Design review of the part shown in the three views and the two pictorial views. Dimensions are in mm from the part's minimum x, y and z. Round coordinates to 2 decimals unless told otherwise and drop trailing zeros. Write each loop counter-clockwise with the first axis right and the second up, starting at its lowest first coordinate (ties: lowest second). Pieces come first, ordered by that corner, then holes. Notation, with made-up numbers: (77, 29.25) - (128, 29.25) arc R21 ccw to (128, 68.25) - close; hole circle Ø5 at (-16.75, 6.25). An arc over 180 degrees is marked (long way). Use one line per item in the form item = value.
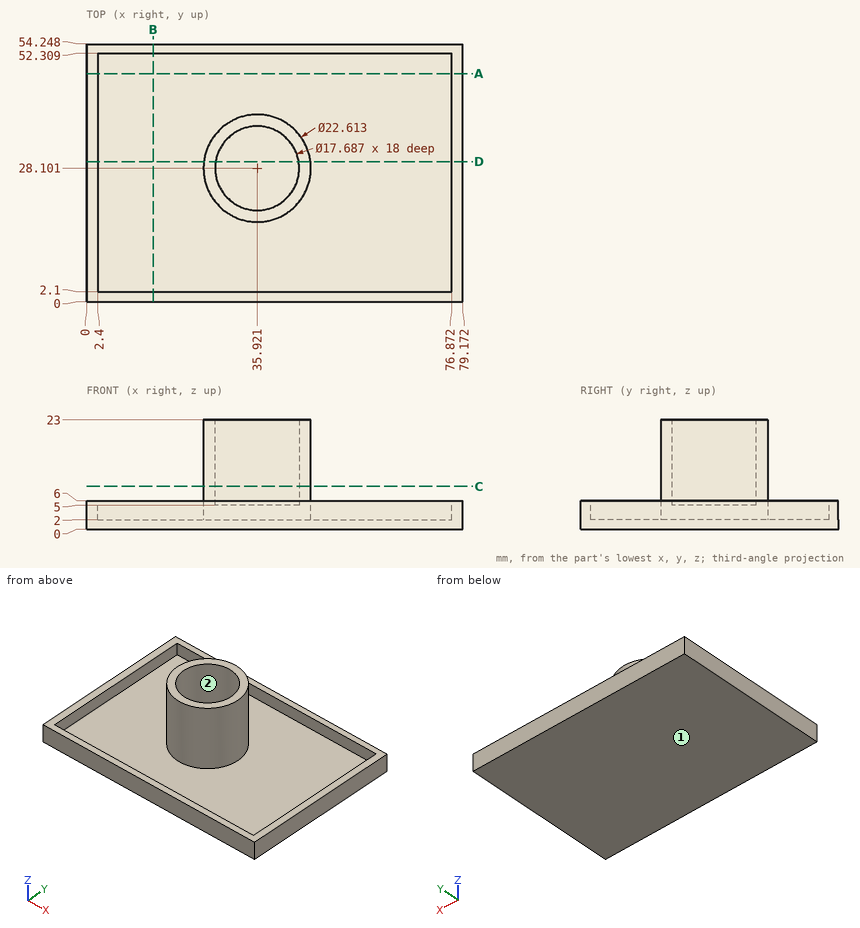
Q1. Draft analysis for pull direction X (two halves, no side actions). For the marked faces 1 and 2, state which applies: released by +X, released by -X, zero draft, split by the parting line, or undercut.
Calculated:
face_1 = zero draft
face_2 = undercut
Q2. To check wall thickness, follow line 1 along X through (y, z) = (28, 19.25) (1 decimal); line 2 along X through (y, z) = (47, 5.75); line 3 along Y through (x, z) = (66, 5). State the ranges of each line that lie inside material, in increasing order. Write a range as from..to.
Calculated:
line_1 = 24.6..27.1, 44.8..47.2
line_2 = 0..2.4, 76.87..79.17
line_3 = 0..2.1, 52.31..54.25
Q3. For P1, Ø12, axis at y = 12, z = 19, coming from the -X side; P2, Ø12, axis at x = 40, z = 19, coming from the -Y side (1 decimal); P3, Ø2, axis at x = 63.5, y = 9.5, coming from the +Z side, all flat-tipped, find the tip position at first contact; note any pin that passes through.
Calculated:
P1 = 30.84
P2 = 16.8
P3 = 2
Q4. We need section D-D on y = 29.5. Write out the cut boundary in (x, z).
Calculated:
outline = (0, 0) - (79.17, 0) - (79.17, 6) - (76.87, 6) - (76.87, 2) - (47.14, 2) - (47.14, 23) - (44.65, 23) - (44.65, 5) - (27.19, 5) - (27.19, 23) - (24.7, 23) - (24.7, 2) - (2.4, 2) - (2.4, 6) - (0, 6) - close
Q5. We need section A-A on y = 48. Write out the cut boundary in (x, z), then the cut area to 3 significant figures.
Calculated:
outline = (0, 0) - (79.17, 0) - (79.17, 6) - (76.87, 6) - (76.87, 2) - (2.4, 2) - (2.4, 6) - (0, 6) - close
area = 177 mm2
Q6. We need section C-C on z = 9. Write out the cut boundary in (x, y) (1 decimal).
Calculated:
outline = circle Ø22.6 at (35.9, 28.1); hole circle Ø17.7 at (35.9, 28.1)
Q7. We need section B-B on x = 14. Write out the cut boundary in (y, z).
Calculated:
outline = (0, 0) - (54.25, 0) - (54.25, 6) - (52.31, 6) - (52.31, 2) - (2.1, 2) - (2.1, 6) - (0, 6) - close
